```python
from build123d import *

# Parameters (mm, degrees)
F0_W         = 77.51
F0_H         = 77.519
F0_R         = 2.55
F0_R_2       = 5
F1_DEPTH     = 16
F2_DEPTH     = 7
F3_R         = 5
F4_R         = 6
F4_R_2       = 2.55
F5_DEPTH     = 4.6
F6_S5_R      = 2.55
F6_T6_DEPTH  = 10
F6_S11_R     = 2.55
F6_T12_DEPTH = 10
F6_S17_R     = 2.55
F6_T18_DEPTH = 10
F6_S23_R     = 2.55
F6_T24_DEPTH = 10


# Not quite as in the source:
# - a fillet or chamfer that OpenCascade refuses, or shapes differently, is made with other operations: its cross-section is extruded or revolved along the edge and cut away or added
# - a feature names something its author has since deleted; it is built from what else it names


with BuildPart() as f1:
    # F0 (on Top) → F1 (new body)
    with BuildSketch(Plane.XY):
        Rectangle(F0_W, F0_H)
        with Locations((-30, -29.9995)):
            Circle(F0_R, mode=Mode.SUBTRACT)
        with Locations((30, -29.9995)):
            Circle(F0_R, mode=Mode.SUBTRACT)
        with Locations((-30, 29.9995)):
            Circle(F0_R, mode=Mode.SUBTRACT)
        Polygon((7.25, -4.1857894516), (0, -8.3715789032), (-7.25, -4.1857894516), (-7.25, 4.1857894516), (0, 8.3715789032), (7.25, 4.1857894516), align=None, mode=Mode.SUBTRACT)
        with Locations((30, 29.9995)):
            Circle(F0_R, mode=Mode.SUBTRACT)
        Polygon((-7.25, -4.1857894516), (0, -8.3715789032), (7.25, -4.1857894516), (7.25, 4.1857894516), (0, 8.3715789032), (-7.25, 4.1857894516), align=None)
        Circle(F0_R_2, mode=Mode.SUBTRACT)
    extrude(amount=F1_DEPTH)

    # F0 (on Top) → F2 (cut)
    with BuildSketch(Plane.XY):
        Polygon((-7.25, -4.1857894516), (0, -8.3715789032), (7.25, -4.1857894516), (7.25, 4.1857894516), (0, 8.3715789032), (-7.25, 4.1857894516), align=None)
        Circle(F0_R_2, mode=Mode.SUBTRACT)
    extrude(amount=F2_DEPTH, mode=Mode.SUBTRACT)

    # F3
    f3_edges = [f1.edges().sort_by_distance(p)[0] for p in [
        (38.755, -38.7595, 8),
        (-38.755, -38.7595, 8),
        (38.755, 38.7595, 8),
        (-38.755, 38.7595, 8),
    ]]
    fillet(f3_edges, radius=F3_R)

    # F4 (on face) → F5 (cut)
    with BuildSketch(Plane.XY.offset(16)):
        with Locations((-30, 29.9995)):
            Circle(F4_R)
        with Locations((-30, 29.9995)):
            Circle(F4_R_2, mode=Mode.SUBTRACT)
        with Locations((30, 29.9995)):
            Circle(F4_R)
        with Locations((30, 29.9995)):
            Circle(F4_R_2, mode=Mode.SUBTRACT)
        with Locations((30, -29.9995)):
            Circle(F4_R)
        with Locations((30, -29.9995)):
            Circle(F4_R_2, mode=Mode.SUBTRACT)
        with Locations((-30, -29.9995)):
            Circle(F4_R)
        with Locations((-30, -29.9995)):
            Circle(F4_R_2, mode=Mode.SUBTRACT)
    extrude(amount=-F5_DEPTH, mode=Mode.SUBTRACT)

    # F6: fillet of radius 3.5 on 4 edges, made by hand


with BuildPart() as f6_tool2:
    # F6_s3 → F6_t4 (revolve)
    with BuildSketch(Plane.XZ.offset(29.9995)):
        with BuildLine():
            ThreePointArc((-24, 14.9), (-25.0251262658, 12.4251262658), (-27.5, 11.4))
            Line((-27.5, 11.4), (-24, 11.4))
            Line((-24, 11.4), (-24, 14.9))
        make_face()
    revolve(axis=Axis((-30, -29.9995, 11.4), (0, 0, 1)))

    # F6_s5 → F6_t6 (cut, symmetric)
    with BuildSketch(Plane.XY.offset(13.2)):
        with Locations((-30, -29.9995)):
            Circle(F6_S5_R)
    extrude(amount=F6_T6_DEPTH, both=True, mode=Mode.SUBTRACT)


with BuildPart() as f1_1:
    add(f1.part)

    # F6_t1: union F6_tool2
    add(f6_tool2.part)


with BuildPart() as f6_tool8:
    # F6_s9 → F6_t10 (revolve)
    with BuildSketch(Plane.XZ.offset(-29.9995)):
        with BuildLine():
            ThreePointArc((-24, 14.9), (-25.0251262658, 12.4251262658), (-27.5, 11.4))
            Line((-27.5, 11.4), (-24, 11.4))
            Line((-24, 11.4), (-24, 14.9))
        make_face()
    revolve(axis=Axis((-30, 29.9995, 11.4), (0, 0, 1)))

    # F6_s11 → F6_t12 (cut, symmetric)
    with BuildSketch(Plane.XY.offset(13.2)):
        with Locations((-30, 29.9995)):
            Circle(F6_S11_R)
    extrude(amount=F6_T12_DEPTH, both=True, mode=Mode.SUBTRACT)


with BuildPart() as f1_2:
    add(f1_1.part)

    # F6_t7: union F6_tool8
    add(f6_tool8.part)


with BuildPart() as f6_tool14:
    # F6_s15 → F6_t16 (revolve)
    with BuildSketch(Plane.XZ.offset(29.9995)):
        with BuildLine():
            ThreePointArc((36, 14.9), (34.9748737342, 12.4251262658), (32.5, 11.4))
            Line((32.5, 11.4), (36, 11.4))
            Line((36, 11.4), (36, 14.9))
        make_face()
    revolve(axis=Axis((30, -29.9995, 11.4), (0, 0, 1)))

    # F6_s17 → F6_t18 (cut, symmetric)
    with BuildSketch(Plane.XY.offset(13.2)):
        with Locations((30, -29.9995)):
            Circle(F6_S17_R)
    extrude(amount=F6_T18_DEPTH, both=True, mode=Mode.SUBTRACT)


with BuildPart() as f1_3:
    add(f1_2.part)

    # F6_t13: union F6_tool14
    add(f6_tool14.part)


with BuildPart() as f6_tool20:
    # F6_s21 → F6_t22 (revolve)
    with BuildSketch(Plane.XZ.offset(-29.9995)):
        with BuildLine():
            ThreePointArc((36, 14.9), (34.9748737342, 12.4251262658), (32.5, 11.4))
            Line((32.5, 11.4), (36, 11.4))
            Line((36, 11.4), (36, 14.9))
        make_face()
    revolve(axis=Axis((30, 29.9995, 11.4), (0, 0, 1)))

    # F6_s23 → F6_t24 (cut, symmetric)
    with BuildSketch(Plane.XY.offset(13.2)):
        with Locations((30, 29.9995)):
            Circle(F6_S23_R)
    extrude(amount=F6_T24_DEPTH, both=True, mode=Mode.SUBTRACT)


with BuildPart() as f1_4:
    add(f1_3.part)

    # F6_t19: union F6_tool20
    add(f6_tool20.part)


solid = f1_4.part
```
The model under review builds one solid part; all positions refer to its coordinate system, in mm. A direction names the side the tool comes from. Round coordinates to 2 decimals unless told otherwise and drop trailing zeros. Order: outer loops, then holes, each group sorted by start corner. A loop starts at its lowest first (then second) coordinate and runs counter-clockwise, first axis right, second up.
Item 1: Machinability: for faces 1 (the flat face through (3.676, 6.249, 3.451)), 2 (the flat face through (-9, 1, 16)), 3 (the cylindrical face through (29.22, 35.95, 15.46)), which of the approach directions +Z, -Z, +X, -X, +Y, -Y give a long, thin tool a straight path to every point of the face, cutting with its end or side? Answer none if there is none.
Working result:
face 1: -Z
face 2: +Z, +X, -X, +Y, -Y
face 3: +Z
Item 2: For pin 1 (4.5 mm diameter, centred on x = -1.5, y = -3, fed in from -Z); pin 2 (6.5 mm diameter, centred on x = 30, y = 30, fed in from +Z), all flat-tipped, find the tip position at first contact; note any pin that passes through.
Working result:
pin 1: stops at z = 7
pin 2: stops at z = 11.48
Item 3: Draft analysis for pull direction Y (two halves, no side actions). For faces 4 (the flat face through (-3.676, -6.249, 3.451)), 5 (the flat face through (38.755, 0, 8)), 6 (the cylindrical face through (-37.329, -37.256, 8.112)), state which applies: released by +Y, released by -Y, zero draft, split by the parting line, or undercut.
Working result:
face 4: undercut
face 5: zero draft
face 6: released by -Y
Item 4: Add section D-D, the plane x = -1.5. State the section outline as (y, z) points.
Working result:
outline: (-38.76, 0) - (-7.51, 0) - (-7.51, 7) - (-4.77, 7) - (-4.77, 16) - (-38.76, 16) - close; (4.77, 7) - (7.51, 7) - (7.51, 0) - (38.76, 0) - (38.76, 16) - (4.77, 16) - close
Item 5: To check wall thickness, follow probe 1 along Y at (x, z) = (30, 7.5); probe 2 along Y at (x, z) = (-30, 15.35); probe 3 along X at (y, z) = (0, 0.75) (3 decimals). State the ranges of each line that lie inside material, in increasing order.
Working result:
probe 1: y = -38.76 to -32.55, -27.45 to 27.45, 32.55 to 38.76
probe 2: y = -38.76 to -36, -24 to 24, 36 to 38.76
probe 3: x = -38.755 to -7.25, 7.25 to 38.755
Item 6: Add section B-B, the plane z = 1. Count the separate pieces of the cut face and the enclosed holes in it, and give its area (3 significant figures).
Working result:
separate pieces: 1
enclosed holes: 5
area: 5,720 mm2
Item 7: Add section A-A, the plane y = 0. State the section outline as (x, z) points (3 decimals), and give its area (3 significant figures).
Working result:
outline: (-38.755, 0) - (-7.25, 0) - (-7.25, 7) - (-5, 7) - (-5, 16) - (-38.755, 16) - close; (5, 7) - (7.25, 7) - (7.25, 0) - (38.755, 0) - (38.755, 16) - (5, 16) - close
area: 1,050 mm2
